Check sheet for the modelled part. Datum: model origin and axes. Units: mm. A direction names the side the tool comes from. Round coordinates to 2 decimals unless told otherwise and drop trailing zeros. Write each loop counter-clockwise with the first axis right and the second up, starting at its lowest first coordinate (ties: lowest second). Pieces come first, ordered by that corner, then holes. Notation, with made-up numbers: M -24.5,73 L 16.5,73 A21 ccw 16.5,102 Z; hole C 70,-35 d6. An arc over 180 degrees is marked long. Answer in a Markdown table with one row per item.
```python
from build123d import *

# Parameters (mm, degrees)
SKETCH2_R           = 10.7696
BOSS_EXTRUDE1_DEPTH = 6.35


with BuildPart() as part:
    # Sketch1 → Revolve1 (revolve)
    with BuildSketch(Plane.XY):
        Polygon((-32.54375, -13.335), (0, -13.335), (0, -7.8994), (-10.31875, -7.8994), (-10.31875, -10.6172), (-32.54375, -10.7696), align=None)
    revolve(axis=Axis((-32.54375, 0, 0), (1, 0, 0)))

    # Sketch2 → Boss-Extrude1 (add)
    with BuildSketch(Plane.ZY.offset(32.54375)):
        Polygon((16.323827371, 0), (11.542689029, 11.542689029), (0, 16.323827371), (-11.542689029, 11.542689029), (-16.323827371, 0), (-11.542689029, -11.542689029), (0, -16.323827371), (11.542689029, -11.542689029), align=None)
        Circle(SKETCH2_R, mode=Mode.SUBTRACT)
    extrude(amount=-BOSS_EXTRUDE1_DEPTH)


solid = part.part
```
1. Section check A-A, the plane x = -6.5. Record the cut outline in (y, z) (3 decimals).
Found:
| item | result |
|---|---|
| outline | C 0,0 d26.67; hole C 0,0 d15.799 |
2. Access from +Z, -Z, +X, -X, +Y, -Y to the whole of each face (thin tool, end or side, straight path). Record for faces 4 (the face through (-10.319, -8, 1)), 5 (the face through (-26.194, 13.4, -2.5)), 6 (the face through (-29.41, -13.9, -5.85)).
Found:
| item | result |
|---|---|
| face 4 | -X |
| face 5 | +X |
| face 6 | -Z, +X, -X, -Y |
3. Go/stop test with flat-tipped pins: pin 1 (1 mm diameter, centred on x = -26.5, z = 3, fed in from +Y); pin 2 (2 mm diameter, centred on x = -19, y = 1, fed in from +Z) (3 decimals); pin 3 (10 mm diameter, centred on x = -3.5, y = 11.5, fed in from +Z). Record where each tip stops, or that it passes through.
Found:
| item | result |
|---|---|
| pin 1 | stops at y = 15.29 |
| pin 2 | stops at z = 13.335 |
| pin 3 | stops at z = 11.64 |
4. Scan lines: L1, parallel to Y at x = -8, z = 0 (3 decimals); L2, parallel to X at y = 10, z = 2. Record each from-to range of solid material in increasing order.
Found:
| item | result |
|---|---|
| L1 | y = -13.335 to -7.899, 7.899 to 13.335 |
| L2 | x = -10.32 to 0 |
5. Section check B-B, the plane x = -27. Record the cut outline in (y, z), and give its area (3 significant figures).
Found:
| item | result |
|---|---|
| outline | M -16.32,0 L -11.54,-11.54 L 0,-16.32 L 11.54,-11.54 L 16.32,0 L 11.54,11.54 L 0,16.32 L -11.54,11.54 Z; hole C 0,0 d21.46 |
| area | 392 mm2 |
6. Draft check along Z on faces 1 (the face through (-32.544, 0, -11)), 2 (the face through (-5.23, 7.89, -0.35)), 3 (the face through (-29.41, -5.85, 13.9)). Enter one of: +Z half, -Z half, draft (parallel to the pull), parting line (faces both ways), or undercut.
Found:
| item | result |
|---|---|
| face 1 | draft |
| face 2 | undercut |
| face 3 | +Z half |
7. Section check C-C, the plane x = -12. Record the cut outline in (y, z) (3 decimals), and give its area (3 significant figures).
Found:
| item | result |
|---|---|
| outline | C 0,0 d26.67; hole C 0,0 d21.257 |
| area | 204 mm2 |
